from build123d import *

# Parameters (mm, degrees)
SCHIZZO1_W                         = 140
SCHIZZO1_H                         = 70
ESTRUSIONE_ESTRUSIONE1_DEPTH       = 3
ESTRUSIONE_ESTRUSIONE2_DEPTH       = 110
SCHIZZO4_W                         = 3
SCHIZZO4_H                         = 19.9
ESTRUSIONE_ESTRUSIONE3_DEPTH       = 140
SCHIZZO5_W                         = 3
SCHIZZO5_H                         = 67
ESTRUSIONE_ESTRUSIONE4_DEPTH       = 89.5
TAGLIO_ESTRUSIONE1_REACH           = 183.814
TAGLIO_ESTRUSIONE3_DEPTH           = 110
RACCORDO1_R                        = 2
SCHIZZO8_R                         = 1.7
TAGLIO_ESTRUSIONE4_DEPTH           = 182.813778356
SCHIZZO10_R                        = 3
TAGLIO_ESTRUSIONE5_DEPTH           = 2
TAGLIO_ESTRUSIONE5_DRAFT           = -45
TAGLIO_ESTRUSIONE5_PROFILE_2_DEPTH = 2
TAGLIO_ESTRUSIONE5_PROFILE_2_DRAFT = -45
SCHIZZO11_R                        = 3
TAGLIO_ESTRUSIONE6_DEPTH           = 2
TAGLIO_ESTRUSIONE6_DRAFT           = -45
TAGLIO_ESTRUSIONE6_PROFILE_2_DEPTH = 2
TAGLIO_ESTRUSIONE6_PROFILE_2_DRAFT = -45
TAGLIO_ESTRUSIONE7_DEPTH           = 3
SCHIZZO13_R                        = 4.15
TAGLIO_ESTRUSIONE8_DEPTH           = 10


with BuildPart() as part:
    # Schizzo1 → Estrusione-Estrusione1 (new body)
    with BuildSketch(Plane(origin=(0, 0, 0), x_dir=(1, 0, 0), z_dir=(0, 1, 0))):
        with Locations((-70, -35)):
            Rectangle(SCHIZZO1_W, SCHIZZO1_H)
    extrude(amount=ESTRUSIONE_ESTRUSIONE1_DEPTH)

    # Schizzo2 → Estrusione-Estrusione2 (add)
    with BuildSketch(Plane(origin=(-15, 0, 0), x_dir=(0, 0, -1), z_dir=(1, 0, 0))):
        Polygon((-8.240628014, 3), (-8.240628014, 19.794228272), (-4.225592959, 25.528292582), (-3, 22.9), (-3, 3), align=None)
    extrude(amount=-ESTRUSIONE_ESTRUSIONE2_DEPTH)

    # Schizzo4 → Estrusione-Estrusione3 (add)
    with BuildSketch(Plane(origin=(0, 0, 0), x_dir=(0, 0, -1), z_dir=(1, 0, 0))):
        with Locations((-1.5, 12.95)):
            Rectangle(SCHIZZO4_W, SCHIZZO4_H)
    extrude(amount=-ESTRUSIONE_ESTRUSIONE3_DEPTH)

    # Schizzo5 → Estrusione-Estrusione4 (add)
    with BuildSketch(Plane(origin=(0, 3, 0), x_dir=(1, 0, 0), z_dir=(0, 1, 0))):
        with Locations((-138.5, -36.5)):
            Rectangle(SCHIZZO5_W, SCHIZZO5_H)
        with Locations((-1.5, -36.5)):
            Rectangle(SCHIZZO5_W, SCHIZZO5_H)
    extrude(amount=ESTRUSIONE_ESTRUSIONE4_DEPTH)

    # Taglio-Estrusione1: up to this face of the body (flat: up to its plane)
    taglio_estrusione1_end = Plane(part.part.faces().sort_by_distance((0, 45.868467333, 36.116274616))[0])
    # Schizzo6 → Taglio-Estrusione1 (cut, up to the picked face)
    with BuildSketch(Plane.ZY.offset(140), mode=Mode.PRIVATE) as taglio_estrusione1_sk1:
        Polygon((3, 23), (35.408382242, 92.5), (3, 92.5), align=None)
    taglio_estrusione1_tool1 = split(extrude(taglio_estrusione1_sk1.sketch, amount=-TAGLIO_ESTRUSIONE1_REACH, mode=Mode.PRIVATE), bisect_by=taglio_estrusione1_end, keep=Keep.BOTH, mode=Mode.PRIVATE)
    add(taglio_estrusione1_tool1.solids().sort_by(Axis((-140, 69.333333, 13.802794), (1, 0, 0)))[0], mode=Mode.SUBTRACT)

    # Schizzo7 → Taglio-Estrusione3 (cut)
    with BuildSketch(Plane.ZY.offset(125)):
        Polygon((61.85, 3), (70, 3), (70, 2.85), (66, 2.85), (66, 0.85), (61.85, 0.85), align=None)
    extrude(amount=-TAGLIO_ESTRUSIONE3_DEPTH, mode=Mode.SUBTRACT)

    # Raccordo1
    raccordo1_edges = [part.edges().sort_by_distance(p)[0] for p in [
        (-140, 0, 35),
        (-70, 0, 0),
        (0, 0, 35),
        (-140, 11.45, 0),
        (0, 11.45, 0),
    ]]
    fillet(raccordo1_edges, radius=RACCORDO1_R)

    # Schizzo8 → Taglio-Estrusione4 (cut, through all)
    with BuildSketch(Plane.ZY.offset(140)):
        with Locations((45, 87.5)):
            Circle(SCHIZZO8_R)
        with Locations((65, 87.5)):
            Circle(SCHIZZO8_R)
    extrude(amount=-TAGLIO_ESTRUSIONE4_DEPTH, mode=Mode.SUBTRACT)


with BuildPart() as taglio_estrusione5_tool:
    # Schizzo10 → Taglio-Estrusione5 (with draft: the straight prism first)
    with BuildSketch(Plane.ZY.offset(140)):
        with Locations((45, 87.5)):
            Circle(SCHIZZO10_R)
    extrude(amount=-TAGLIO_ESTRUSIONE5_DEPTH)
    # Taglio-Estrusione5: the draft: its side faces are tilted about the plane it starts from
    taglio_estrusione5_sides = [taglio_estrusione5_tool.faces().sort_by_distance(p)[0] for p in [
        (-139, 87.5, 42),
    ]]
    draft(taglio_estrusione5_sides, Plane.ZY.offset(140), TAGLIO_ESTRUSIONE5_DRAFT)


with BuildPart() as part_1:
    add(part.part)

    # Taglio-Estrusione5: cut by taglio_estrusione5_tool
    add(taglio_estrusione5_tool.part, mode=Mode.SUBTRACT)


with BuildPart() as taglio_estrusione5_profile_2_tool:
    # Schizzo10 → Taglio-Estrusione5 profile 2 (with draft: the straight prism first)
    with BuildSketch(Plane.ZY.offset(140)):
        with Locations((65, 87.5)):
            Circle(SCHIZZO10_R)
    extrude(amount=-TAGLIO_ESTRUSIONE5_PROFILE_2_DEPTH)
    # Taglio-Estrusione5 profile 2: the draft: its side faces are tilted about the plane it starts from
    taglio_estrusione5_profile_2_sides = [taglio_estrusione5_profile_2_tool.faces().sort_by_distance(p)[0] for p in [
        (-139, 87.5, 62),
    ]]
    draft(taglio_estrusione5_profile_2_sides, Plane.ZY.offset(140), TAGLIO_ESTRUSIONE5_PROFILE_2_DRAFT)


with BuildPart() as part_2:
    add(part_1.part)

    # Taglio-Estrusione5 profile 2: cut by taglio_estrusione5_profile_2_tool
    add(taglio_estrusione5_profile_2_tool.part, mode=Mode.SUBTRACT)


with BuildPart() as taglio_estrusione6_tool:
    # Schizzo11 → Taglio-Estrusione6 (with draft: the straight prism first)
    with BuildSketch(Plane(origin=(0, 0, 0), x_dir=(0, 0, -1), z_dir=(1, 0, 0))):
        with Locations((-65, 87.5)):
            Circle(SCHIZZO11_R)
    extrude(amount=-TAGLIO_ESTRUSIONE6_DEPTH)
    # Taglio-Estrusione6: the draft: its side faces are tilted about the plane it starts from
    taglio_estrusione6_sides = [taglio_estrusione6_tool.faces().sort_by_distance(p)[0] for p in [
        (-1, 87.5, 68),
    ]]
    draft(taglio_estrusione6_sides, Plane(origin=(0, 0, 0), x_dir=(0, 0, -1), z_dir=(1, 0, 0)), TAGLIO_ESTRUSIONE6_DRAFT)


with BuildPart() as part_3:
    add(part_2.part)

    # Taglio-Estrusione6: cut by taglio_estrusione6_tool
    add(taglio_estrusione6_tool.part, mode=Mode.SUBTRACT)


with BuildPart() as taglio_estrusione6_profile_2_tool:
    # Schizzo11 → Taglio-Estrusione6 profile 2 (with draft: the straight prism first)
    with BuildSketch(Plane(origin=(0, 0, 0), x_dir=(0, 0, -1), z_dir=(1, 0, 0))):
        with Locations((-45, 87.5)):
            Circle(SCHIZZO11_R)
    extrude(amount=-TAGLIO_ESTRUSIONE6_PROFILE_2_DEPTH)
    # Taglio-Estrusione6 profile 2: the draft: its side faces are tilted about the plane it starts from
    taglio_estrusione6_profile_2_sides = [taglio_estrusione6_profile_2_tool.faces().sort_by_distance(p)[0] for p in [
        (-1, 87.5, 48),
    ]]
    draft(taglio_estrusione6_profile_2_sides, Plane(origin=(0, 0, 0), x_dir=(0, 0, -1), z_dir=(1, 0, 0)), TAGLIO_ESTRUSIONE6_PROFILE_2_DRAFT)


with BuildPart() as part_4:
    add(part_3.part)

    # Taglio-Estrusione6 profile 2: cut by taglio_estrusione6_profile_2_tool
    add(taglio_estrusione6_profile_2_tool.part, mode=Mode.SUBTRACT)

    # Schizzo12 → Taglio-Estrusione7 (cut)
    with BuildSketch(Plane.ZY.offset(140)):
        with BuildLine():
            Line((37.724413642, 20.258722006), (42.5, 30.5))
            ThreePointArc((42.5, 30.5), (42.545069526, 31.532261847), (41.847019141, 32.294050166))
            Line((41.847019141, 32.294050166), (36.409172419, 34.829759736))
            ThreePointArc((36.409172419, 34.829759736), (35.376910572, 34.874829262), (34.615122253, 34.176778877))
            Line((34.615122253, 34.176778877), (29.839535895, 23.935500884))
            ThreePointArc((29.839535895, 23.935500884), (29.79446637, 22.903239037), (30.492516754, 22.141450718))
            Line((30.492516754, 22.141450718), (35.930363476, 19.605741147))
            ThreePointArc((35.930363476, 19.605741147), (36.962625323, 19.560671622), (37.724413642, 20.258722006))
        make_face()
    extrude(amount=-TAGLIO_ESTRUSIONE7_DEPTH, mode=Mode.SUBTRACT)

    # Schizzo13 → Taglio-Estrusione8 (cut)
    with BuildSketch(Plane.ZY.offset(140)):
        with Locations((57, 20)):
            Circle(SCHIZZO13_R)
    extrude(amount=-TAGLIO_ESTRUSIONE8_DEPTH, mode=Mode.SUBTRACT)


solid = part_4.part
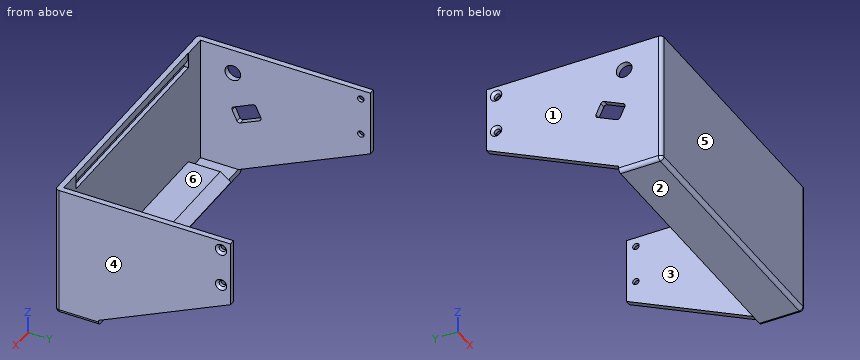
Check sheet for the modelled part. Datum: model origin and axes. Units: mm. Face numbers are marked on the shaded views. A direction names the side the tool comes from. Give positions to 0.01 mm unless a question says otherwise; leave off trailing zeros. Order: outer loops, then holes, each group sorted by start corner. A loop starts at its lowest first (then second) coordinate and runs counter-clockwise, first axis right, second up. Notation, with made-up numbers: M 44.5,79.5 L 82.5,79.5 A26 ccw 82.5,104.5 Z; hole C 15.5,57 d1. An arc over 180 degrees is marked long. Answer as CSV lines item,"result". Start each with the question number.
Item 1: Cross-section at C-C on x = -110.5. Enter the section's corners in (y, z).
Item 2: Cross-section at D-D on y = 87.5. State how many separate pieces and enclosed holes the cut face has, plus the area to 3 significant figures.
Item 3: Gauge pin test, flat ends, axial feed: P1, Ø3.5, axis at x = -79.5, z = 63.5, coming from the +Y side; P2, Ø2.5, axis at x = -104.5, z = 1.5, coming from the +Y side; P3, Ø5, axis at x = -62.5, y = 9.5, coming from the +Z side. Record the tip position at first contact, or that the pin passes through.
Item 4: Mould release check, pull along X, two halves, no side actions. Record for the marked faces 1, 2, 3 and 4: +X half, -X half, draft (parallel to the pull), parting line (faces both ways), or undercut.
Item 5: Thickness scan on line 1 (X direction, y = 9, z = 8.5); line 2 (Y direction, x = -2.6, z = 65); line 3 (Z direction, x = -138.2, y = 87.5). Record the ranges inside material, lowest first. Write a range as [from, to].
Item 6: Cross-section at B-B on y = 37.5. Enter the section's corners in (x, z).
Item 7: Tool access check on the marked faces 5 and 6. Record the directions out of +Z, -Z, +X, -X, +Y, -Y that give a thin tool (end or side, any length) a straight path to the whole face; none if there is none.
Item 8: Cross-section at A-A on z = 57. Enter the section's corners in (x, y).
Established:
1,outline,"M 0,2 A2 ccw 2,0 L 22.9,0 L 22.9,3 L 25.53,4.23 L 19.79,8.24 L 3,8.24 L 3,61.85 L 0.85,61.85 L 0.85,66 L 2.85,66 L 2.85,70 L 0,70 Z"
2,separate pieces,"6"
2,enclosed holes,"0"
2,area,"174 mm^2"
3,P1,"stops at y = 3"
3,P2,"stops at y = 22.9"
3,P3,"stops at z = 8.24"
4,face 1,"-X half"
4,face 2,"draft"
4,face 3,"undercut"
4,face 4,"+X half"
5,line 1,"x = [-140, -137], [-3, 0]"
5,line 2,"y = [0, 85.8], [89.2, 92.5]"
5,line 3,"z = [33.08, 43.3], [46.7, 63.3], [66.7, 70]"
6,outline,"M -140,9.76 L -137,9.76 L -137,70 L -140,70 Z; M -3,9.76 L 0,9.76 L 0,70 L -3,70 Z"
7,face 5,"+Z, -Z, +X, -X, -Y"
7,face 6,"+Z, +Y"
8,outline,"M -140,2 A2 ccw -138,0 L -2,0 A2 ccw 0,2 L 0,92.5 L -3,92.5 L -3,3 L -137,3 L -137,15.85 L -140,15.85 Z; M -140,24.15 L -137,24.15 L -137,92.5 L -140,92.5 Z"
